Verification items for the finished model (mm, model axes). Face numbers are marked on the shaded views. A direction names the side the tool comes from. Coordinates: 2 decimals unless noted, no trailing zeros. Order: outer loops, then holes, each group sorted by start corner. A loop starts at its lowest first (then second) coordinate and runs counter-clockwise, first axis right, second up.
Q1. Depth check by flat-ended pin: P1, Ø4, axis at y = 6.5, z = 17.5, coming from the -X side; P2, Ø5, axis at x = -8, z = -1, coming from the +Y side; P3, Ø1, axis at y = 16, z = 23.5, coming from the -X side; P4, Ø10, axis at y = 26.5, z = -8, coming from the +X side. Enter the tip coordinate at first touch or a pass-through.
Q2. Thickness scan on line 1 (Y direction, x = 13.5, z = 26); line 2 (X direction, y = 26, z = 0); line 3 (Z direction, x = 2.5, y = 22.5). Record the ranges inside material, lowest first.
Q3. Cross-section at A-A, the plane x = 0. Record the boundary of the cut face in (y, z).
Q4. Cross-section at C-C, the plane x = 24.5. Record the boundary of the cut face in (y, z), and give its area (3 significant figures).
Q5. Cross-section at B-B, the plane z = 0. Record the boundary of the cut face in (x, y), and give its area (3 significant figures).
Q6. Cross-section at D-D, the plane y = 7. Record the boundary of the cut face in (x, z).
Q7. Draft check along X on the marked faces 1, 2 and 3. Enter one of: pulls with the +X half, pulls with the -X half, needs draft (parallel to the pull), parting line crosses it, or undercut.
Q8. Set-up check for the marked faces 4 and 5: record each of +Z, -Z, +X, -X, +Y, -Y from which the full face is reachable in a straight line by a thin tool's end or side.
from build123d import *

# Parameters (mm, degrees)
SKETCH_1_R             = 30
SKETCH_1_R_2           = 12.5
EXTRUDE_1_DEPTH        = 34
CUT_EXTRUDE_START      = -6
SKETCH_2_R             = 30
SKETCH_2_R_2           = 28
CUT_EXTRUDE_1_DEPTH    = 6
PATTERN_LINEAR_1_COUNT = 3
PATTERN_LINEAR_1_PITCH = 14


with BuildPart() as part:
    # 草图1 → 凸台-拉伸1 (new body)
    with BuildSketch(Plane(origin=(0, 0, 0), x_dir=(1, 0, 0), z_dir=(0, 1, 0))):
        with Locations(Location((0, 0, 0), (0, 0, 270))):
            Circle(SKETCH_1_R)
        with Locations(Location((0, 0, 0), (0, 0, 270))):
            Circle(SKETCH_1_R_2, mode=Mode.SUBTRACT)
    extrude(amount=EXTRUDE_1_DEPTH)

    # 草图2 → 切除-拉伸1 (cut)
    with BuildSketch(Plane(origin=(0, 34, 0), x_dir=(1, 0, 0), z_dir=(0, 1, 0)).offset(CUT_EXTRUDE_START)):
        with Locations(Location((0, 0, 0), (0, 0, 270))):
            Circle(SKETCH_2_R)
        with Locations(Location((0, 0, 0), (0, 0, 270))):
            Circle(SKETCH_2_R_2, mode=Mode.SUBTRACT)
    cut_extrude_1 = extrude(amount=CUT_EXTRUDE_1_DEPTH, mode=Mode.SUBTRACT)

    # 阵列(线性)1: 切除-拉伸1 ×3
    with Locations(*[(0, -i * PATTERN_LINEAR_1_PITCH, 0) for i in range(1, PATTERN_LINEAR_1_COUNT)]):
        add(cut_extrude_1, mode=Mode.SUBTRACT)


solid = part.part
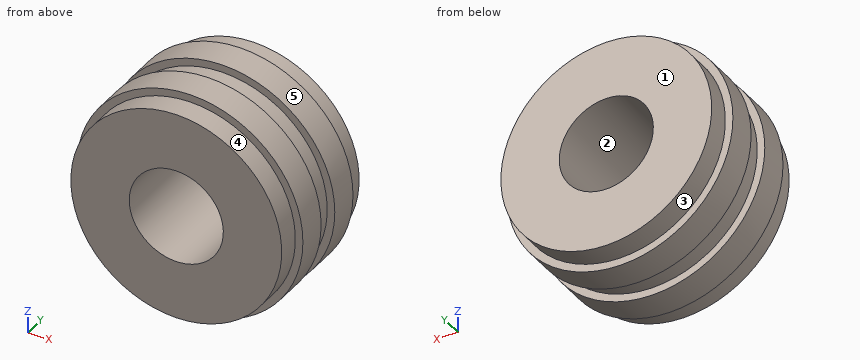
Check values:
1. P1: stops at x = -25.69
1. P2: passes through
1. P3: stops at x = -15.97
1. P4: stops at x = 29.85
2. line 1: y = 6 to 14, 20 to 28
2. line 2: x = -30 to -12.5, 12.5 to 30
2. line 3: z = -29.9 to -12.25, 12.25 to 29.9
3. outline: (0, -28) - (6, -28) - (6, -30) - (14, -30) - (14, -28) - (20, -28) - (20, -30) - (28, -30) - (28, -28) - (34, -28) - (34, -12.5) - (0, -12.5) - close; (0, 12.5) - (34, 12.5) - (34, 28) - (28, 28) - (28, 30) - (20, 30) - (20, 28) - (14, 28) - (14, 30) - (6, 30) - (6, 28) - (0, 28) - close
4. outline: (0, -13.56) - (6, -13.56) - (6, -17.31) - (14, -17.31) - (14, -13.56) - (20, -13.56) - (20, -17.31) - (28, -17.31) - (28, -13.56) - (34, -13.56) - (34, 13.56) - (28, 13.56) - (28, 17.31) - (20, 17.31) - (20, 13.56) - (14, 13.56) - (14, 17.31) - (6, 17.31) - (6, 13.56) - (0, 13.56) - close
4. area: 1,040 mm2
5. outline: (-30, 6) - (-28, 6) - (-28, 0) - (-12.5, 0) - (-12.5, 34) - (-28, 34) - (-28, 28) - (-30, 28) - (-30, 20) - (-28, 20) - (-28, 14) - (-30, 14) - close; (12.5, 0) - (28, 0) - (28, 6) - (30, 6) - (30, 14) - (28, 14) - (28, 20) - (30, 20) - (30, 28) - (28, 28) - (28, 34) - (12.5, 34) - close
5. area: 1,120 mm2
6. outline: circle Ø60 at (0, 0); hole circle Ø25 at (0, 0)
7. face 1: needs draft
7. face 2: undercut
7. face 3: parting line crosses it
8. face 4: -Y
8. face 5: +Y, -Y
